Geometry check sheet. Reference: the model listing, model coordinates, mm. Round coordinates to 2 decimals unless told otherwise and drop trailing zeros. Order: outer loops, then holes, each group sorted by start corner. A loop starts at its lowest first (then second) coordinate and runs counter-clockwise, first axis right, second up.
(1) Cross-section at A-A on y = 21.25. Count the separate pieces of the cut face and the enclosed holes in it, and give its area (3 significant figures).
(2) Cross-section at B-B on x = -58. Enter the section's corners in (y, z).
(3) Cross-section at C-C on z = -17.5. Enter the section's corners in (x, y), and give its area (3 significant figures).
(4) Thickness scan on L1, parallel to X at y = 31.25, z = -37.5; L2, parallel to Z at x = -60, y = 10.5; L3, parallel to Z at x = -71, y = 14.75. Record the ranges inside material, lowest first.
(5) Gauge pin test, flat ends, axial feed: P1, Ø1.5, axis at x = -67.5, y = 24, coming from the -Z side; P2, Ø5, axis at x = -48.5, y = 29.5, coming from the -Z side; P3, Ø5, axis at x = -53.49, y = 27, coming from the +Z side. Record the tip position at first contact, or that the pin passes through.
from build123d import *

# Parameters (mm, degrees)
SKETCH103_W             = 27
SKETCH103_H             = 27
SKETCH103_R             = 1.5
PAD047_DEPTH            = 3
SKETCH102_R             = 11.5
SKETCH102_R_2           = 1.6
PAD048_DEPTH            = 3
PAD049_DEPTH            = 27
BODY011_ROLL_ANGLE      = -89.982677
BODY011_PITCH_ANGLE     = -0.017318
BODY011_PLACEMENT_ANGLE = 89.982677


with BuildPart() as part:
    # Sketch103 → Pad047 (new body)
    with BuildSketch(Plane.XZ):
        with Locations((13.5, -13.5)):
            Rectangle(SKETCH103_W, SKETCH103_H)
        with Locations((7, -16.5)):
            Circle(SKETCH103_R, mode=Mode.SUBTRACT)
        with Locations((13.5, -19.5)):
            Circle(SKETCH103_R, mode=Mode.SUBTRACT)
        with Locations((20, -16.5)):
            Circle(SKETCH103_R, mode=Mode.SUBTRACT)
    extrude(amount=-PAD047_DEPTH)

    # Sketch102 → Pad048 (join)
    with BuildSketch(Plane.XY):
        with BuildLine():
            Line((0, 42), (0, 0))
            Line((0, 0), (27, 0))
            Line((27, 0), (27, 42))
            ThreePointArc((27, 42), (26.12132, 44.12132), (24, 45))
            Line((24, 45), (3, 45))
            ThreePointArc((3, 45), (0.87868, 44.12132), (0, 42))
        make_face()
        with Locations((13.5, 29.5)):
            Circle(SKETCH102_R, mode=Mode.SUBTRACT)
        with Locations((3.8, 39.2)):
            Circle(SKETCH102_R_2, mode=Mode.SUBTRACT)
        with Locations((23.2, 39.2)):
            Circle(SKETCH102_R_2, mode=Mode.SUBTRACT)
        with Locations((23.2, 19.8)):
            Circle(SKETCH102_R_2, mode=Mode.SUBTRACT)
        with Locations((3.8, 19.8)):
            Circle(SKETCH102_R_2, mode=Mode.SUBTRACT)
    extrude(amount=PAD048_DEPTH)

    # Sketch104 → Pad049 (join)
    with BuildSketch(Plane.YZ):
        with BuildLine():
            ThreePointArc((10, 0), (2.928931, -2.928933), (0, -10.000003))
            Line((0, -10.000003), (0, 0))
            Line((10, 0), (0, 0))
        make_face()
    extrude(amount=PAD049_DEPTH)


with BuildPart() as part_1:
    # Body011 roll: moved
    add(part.part.rotate(Axis((0, 0, 0), (1, 0, 0)), BODY011_ROLL_ANGLE))


with BuildPart() as part_2:
    # Body011 pitch: moved
    add(part_1.part.rotate(Axis((0, 0, 0), (0, 1, 0)), BODY011_PITCH_ANGLE))


with BuildPart() as part_3:
    # Body011 placement: moved
    add(part_2.part.moved(Location((-70, 7, 0))).rotate(Axis((-70, 7, 0), (0, 0, 1)), BODY011_PLACEMENT_ANGLE))


solid = part_3.part
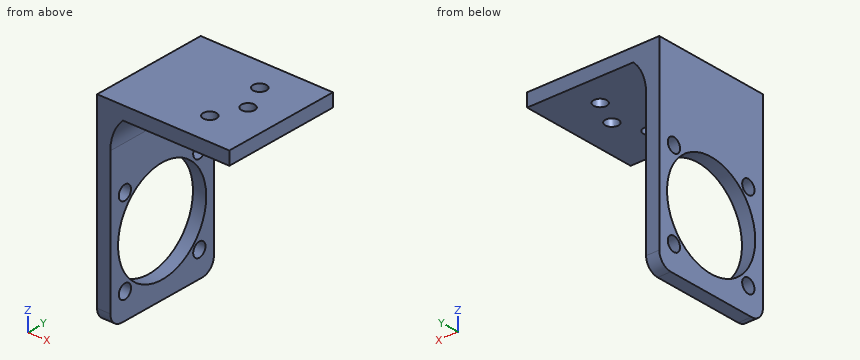
Found:
1. separate pieces: 3
1. enclosed holes: 0
1. area: 146 mm2
2. outline: (7, -3) - (34, -3) - (34, 0) - (7, 0) - close
3. outline: (-73.01, 7.01) - (-70.01, 7.01) - (-70, 34.01) - (-73, 34.01) - close
3. area: 81.0 mm2
4. L1: x = -73 to -70
4. L2: z = -3 to 0
4. L3: z = -45 to -39.45, -19.54 to 0
5. P1: stops at z = -4.35
5. P2: stops at z = -3
5. P3: stops at z = 0
